Geometry check sheet. Reference: the model listing, model coordinates, mm. A direction names the side the tool comes from. Give positions to 0.01 mm unless a question says otherwise; leave off trailing zeros. Write each loop counter-clockwise with the first axis right and the second up, starting at its lowest first coordinate (ties: lowest second). Pieces come first, ordered by that corner, then holes. Notation, with made-up numbers: M 47.25,7 L 53.25,7 A37 ccw 53.25,46 Z; hole C 17.5,-36.75 d2. An arc over 180 degrees is marked long. Use one line per item in the form item = value. Start each with the question number.
```python
from build123d import *

# Parameters (mm, degrees)
SKETCH1_R           = 22.225
BOSS_EXTRUDE1_DEPTH = 2.54
SKETCH2_R           = 8.89
BOSS_EXTRUDE2_DEPTH = 13.97
FILLET1_R           = 0.635


with BuildPart() as part:
    # Sketch1 → Boss-Extrude1 (new body)
    with BuildSketch(Plane(origin=(0, 0, 0), x_dir=(1, 0, 0), z_dir=(0, 1, 0))):
        with Locations(Location((0, 0, 0), (0, 0, 270))):
            Circle(SKETCH1_R)
        Polygon((7.478995387, 0), (3.739497694, 6.477), (-3.739497694, 6.477), (-7.478995387, 0), (-3.739497694, -6.477), (3.739497694, -6.477), align=None, mode=Mode.SUBTRACT)
    extrude(amount=BOSS_EXTRUDE1_DEPTH)

    # Sketch2 → Boss-Extrude2 (add)
    with BuildSketch(Plane(origin=(0, 2.54, 0), x_dir=(1, 0, 0), z_dir=(0, 1, 0))):
        with Locations(Location((0, 0, 0), (0, 0, 270))):
            Circle(SKETCH2_R)
        Polygon((3.739497694, 6.477), (-3.739497694, 6.477), (-7.478995387, 0), (-3.739497694, -6.477), (3.739497694, -6.477), (7.478995387, 0), align=None, mode=Mode.SUBTRACT)
    extrude(amount=BOSS_EXTRUDE2_DEPTH)

    # Fillet1
    fillet1_edges = [part.edges().sort_by_distance(p)[0] for p in [
        (0, 0, -6.477),
        (-5.60924654, 0, -3.2385),
        (-5.60924654, 0, 3.2385),
        (0, 0, 6.477),
        (0, 0, -22.225),
        (0, 2.54, -8.89),
        (0, 2.54, -22.225),
        (5.60924654, 0, 3.2385),
        (5.60924654, 0, -3.2385),
    ]]
    fillet(fillet1_edges, radius=FILLET1_R)


solid = part.part
```
(1) Depth check by flat-ended pin: pin 1 (6 mm diameter, centred on y = 4.5, z = -6, fed in from -X); pin 2 (6 mm diameter, centred on x = 1, y = 12, fed in from +Z); pin 3 (6 mm diameter, centred on x = 7.5, y = 7.5, fed in from +Z); pin 4 (12 mm diameter, centred on x = -4.5, z = -4, fed in from -Y). Enter the tip coordinate at first touch or a pass-through.
(2) Draft check along Z on faces 4 (the cylindrical face through (18.74, 1.26, 11.95)), 5 (the flat face through (-5.635, 8.461, 3.193)), 6 (the flat face through (0, 0, 9)). Enter one of: released by +Z, released by -Z, zero draft, split by the parting line, or undercut.
(3) Sectioned sample at B-B, the plane y = 13. Record the boundary of the cut face in (x, z), plus the area to 3 significant figures.
(4) Thickness scan on probe 1 along Y at (x, z) = (-7, 10.5); probe 2 along X at (y, z) = (9.5, 1); probe 3 along Z at (x, y) = (5, 1). Record the ranges inside material, lowest first. Write a range as [from, to].
(5) Tool access check on faces 1 (the flat face through (0, 8, -6.477)), 2 (the cylindrical face through (-5.75, 0.18, 3.38)), 3 (the cylindrical face through (-8.68, 9.75, -1.93)). Record the directions out of +Z, -Z, +X, -X, +Y, -Y that give a thin tool (end or side, any length) a straight path to the whole face; none if there is none.
(6) Sectioned sample at A-A, the plane x = 0. Record the boundary of the cut face in (y, z) (3 decimals).
Numbers:
q1.pin_1 = -21.79
q1.pin_2 = 8.89
q1.pin_3 = 7.67
q1.pin_4 = 0
q2.face_4 = split by the parting line
q2.face_5 = undercut
q2.face_6 = zero draft
q3.outline = C 0,0 d17.78; hole M -7.48,0 L -3.74,-6.48 L 3.74,-6.48 L 7.48,0 L 3.74,6.48 L -3.74,6.48 Z
q3.area = 103 mm2
q4.probe_1 = [0, 2.54]
q4.probe_2 = [-8.83, -6.9], [6.9, 8.83]
q4.probe_3 = [-21.66, -4.29], [4.29, 21.66]
q5.face_1 = +Y, -Y
q5.face_2 = -Y
q5.face_3 = +Y
q6.outline = M 0,-21.59 A0.635 ccw 0.635,-22.225 L 1.905,-22.225 A0.635 ccw 2.54,-21.59 L 2.54,-9.525 A0.635 cw 3.175,-8.89 L 16.51,-8.89 L 16.51,-6.477 L 0.635,-6.477 A0.635 ccw 0,-7.112 Z; M 0,7.112 A0.635 ccw 0.635,6.477 L 16.51,6.477 L 16.51,8.89 L 3.175,8.89 A0.635 cw 2.54,9.525 L 2.54,21.59 A0.635 ccw 1.905,22.225 L 0.635,22.225 A0.635 ccw 0,21.59 Z
